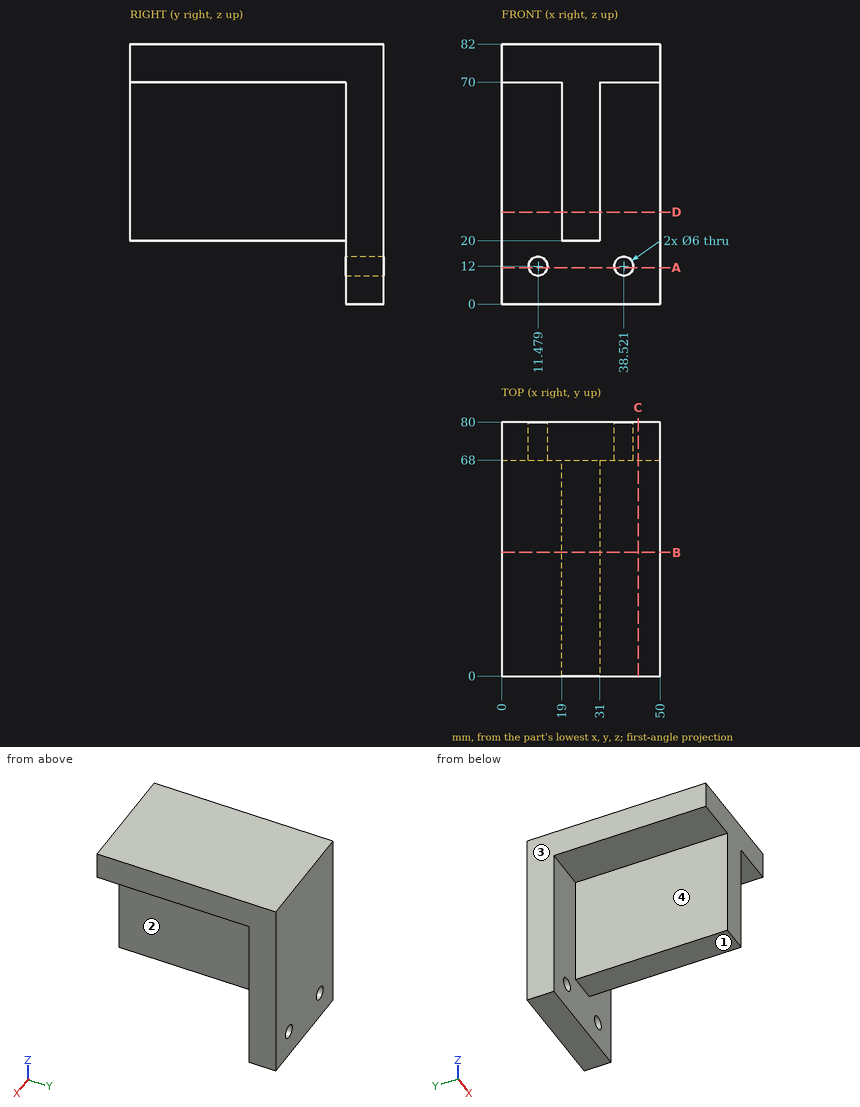
Could you check a few things on this drawing? It's one solid part, dimensions in mm from its lowest x, y, z. A direction names the side the tool comes from. Give positions to 0.01 mm unless a question says otherwise; leave off trailing zeros. Order: outer loops, then holes, each group sorted by start corner. A loop starts at its lowest first (then second) coordinate and runs counter-clockwise, first axis right, second up. Notation, with made-up numbers: (20.5, 10.5) - (69.5, 10.5) arc R9 ccw to (69.5, 26.5) - close; hole circle Ø8 at (-34, 79). An arc over 180 degrees is marked (long way). Answer as a JSON object with one key per item and string values. Group by question number.
Item 1: If we section it at A-A on z = 11.5: Please give me the cut outline in (x, y), and give its area (3 significant figures).
Item 2: Which directions (+Z, -Z, +X, -X, +Y, -Y) give clear straight access to the entire face, cutting with the end or side of a thin tool? Please do the marked faces 1, 2, 3 and 4.
Item 3: If we section it at B-B on y = 39: Please give me the cut outline in (x, z), and give its area (3 significant figures).
Item 4: If we section it at D-D on z = 29: Please give me the cut outline in (x, y), and give its area (3 significant figures).
Item 5: If we section it at C-C on x = 43: Please give me the cut outline in (y, z).
Item 6: Please list where these lines run through material, in increasing order: probe 1 along X at (y, z) = (73, 12); probe 2 along Y at (x, z) = (12, 29); probe 3 along X at (y, z) = (11.5, 56.5).
Item 7: For P1, Ø9.5, axis at x = 25.5, y = 23.5, coming from the -Z side; P2, Ø2, axis at y = 51, z = 25.5, coming from the -X side; P3, Ø5.5, axis at x = 37, y = 24, coming from the -Z side, each with a flat end and sliding along its axis, tell me the tip position at first contact or that it passes through.
Result set:
{
 "1": {"outline": "(0, 68) - (8.52, 68) - (8.52, 80) - (0, 80) - close; (14.44, 68) - (35.56, 68) - (35.56, 80) - (14.44, 80) - close; (41.48, 68) - (50, 68) - (50, 80) - (41.48, 80) - close", "area": "458 mm²"},
 "2": {"face 1": "-Z, +X, -X, -Y", "face 2": "-Z, +X, -Y", "face 3": "+Z, -Z, -X, +Y, -Y", "face 4": "-Z, -X, -Y"},
 "3": {"outline": "(0, 70) - (19, 70) - (19, 20) - (31, 20) - (31, 70) - (50, 70) - (50, 82) - (0, 82) - close", "area": "1,200 mm²"},
 "4": {"outline": "(0, 68) - (19, 68) - (19, 0) - (31, 0) - (31, 68) - (50, 68) - (50, 80) - (0, 80) - close", "area": "1,420 mm²"},
 "5": {"outline": "(0, 70) - (68, 70) - (68, 0) - (80, 0) - (80, 82) - (0, 82) - close"},
 "6": {"probe 1": "0 to 8.48, 14.48 to 35.52, 41.52 to 50", "probe 2": "68 to 80", "probe 3": "19 to 31"},
 "7": {"P1": "z = 20", "P2": "x = 19", "P3": "z = 70"}
}
